Autodesk Inventor part; units mm, degrees
ref_plane "Work Plane1" through (49.8, -24.875, -24.875) normal (1, 0, 0) x (0, 1, 0)
ref_plane "YZ Plane" through (0, 0, 0) normal (1, 0, 0) x (0, 1, 0)
ref_plane "XZ Plane" through (0, 0, 0) normal (0, 1, 0) x (-1, 0, 0)
sketch "Sketch1" plane through (0, 0, 0) normal (1, 0, 0) x (0, 1, 0)
  circle A0 centre (-21.9, 21.9) radius 1.875
  circle A1 centre (21.9, -21.9) radius 1.875
  circle A2 centre (-21.9, -21.9) radius 1.875
  circle A3 centre (21.9, 21.9) radius 1.875
  circle A4 centre (20.8, -14.4) radius 2.0734
  circle A5 centre (-20.8, 14.4) radius 2.0734
  circle A6 centre (-20.8, -14.4) radius 2.0734
  circle A7 centre (-14.4, -20.8) radius 2.0734
  line L0 (17.05, 17.05) -> (-17.05, 17.05)
  line L1 (17.05, -17.05) -> (17.05, 17.05)
  line L2 (-17.05, -17.05) -> (17.05, -17.05)
  line L3 (-17.05, 17.05) -> (-17.05, -17.05)
  circle A8 centre (14.4, -20.8) radius 2.0734
  circle A9 centre (20.8, 14.4) radius 2.0734
  circle A10 centre (-14.4, 20.8) radius 2.0734
  circle A11 centre (14.4, 20.8) radius 2.0734
  line L4 (24.875, 22.9) -> (24.875, -22.9)
  arc A12 (24.875, 22.9) -> (22.9, 24.875) centre (22.9, 22.9) ccw
  line L5 (-22.9, 24.875) -> (22.9, 24.875)
  arc A13 (-22.9, 24.875) -> (-24.875, 22.9) centre (-22.9, 22.9) ccw
  line L6 (-24.875, -22.9) -> (-24.875, 22.9)
  arc A14 (-24.875, -22.9) -> (-22.9, -24.875) centre (-22.9, -22.9) ccw
  line L7 (22.9, -24.875) -> (-22.9, -24.875)
  arc A15 (22.9, -24.875) -> (24.875, -22.9) centre (22.9, -22.9) ccw
  arc A16 (-24.625, -22.9) -> (-22.9, -24.625) centre (-22.9, -22.9) ccw
  line L8 (-24.625, -22.9) -> (-24.625, 22.9)
  arc A17 (-22.9, 24.625) -> (-24.625, 22.9) centre (-22.9, 22.9) ccw
  line L9 (-22.9, 24.625) -> (22.9, 24.625)
  arc A18 (24.625, 22.9) -> (22.9, 24.625) centre (22.9, 22.9) ccw
  line L10 (24.625, 22.9) -> (24.625, -22.9)
  arc A19 (22.9, -24.625) -> (24.625, -22.9) centre (22.9, -22.9) ccw
  line L11 (22.9, -24.625) -> (-22.9, -24.625)
  point P0 (0, 0)
  dimension "d0" = 0.25
ref_plane "Work Plane1" through (49.8, -24.875, -24.875) normal (1, 0, 0) x (0, 1, 0)
extrude "Extrusion1" add sketch "Sketch1" along normal blind 2.5 from surface at 49.8 contours A0 | A1 | A2 | A3 | A4 | A5 | A6 | A7 | L1 L2 L3 L0 | A8 | A9 | A10 | A11 | L8 A17 L9 A18 L10 A19 L11 A16
sketch "Sketch2" plane through (52.3, -22.9, -24.625) normal (1, 0, 0) x (0, 0, -1)
  circle A0 centre (-46.525, 1) radius 1.875
  circle A1 centre (-2.725, 44.8) radius 1.875
  circle A2 centre (-2.725, 1) radius 1.875
  circle A3 centre (-46.525, 44.8) radius 1.875
  circle A4 centre (-10.225, 43.7) radius 2.0734
  circle A5 centre (-39.025, 2.1) radius 2.0734
  circle A6 centre (-10.225, 2.1) radius 2.0734
  circle A7 centre (-3.825, 8.5) radius 2.0734
  line L0 (-41.675, 39.95) -> (-41.675, 5.85)
  line L1 (-7.575, 39.95) -> (-41.675, 39.95)
  line L2 (-7.575, 5.85) -> (-7.575, 39.95)
  line L3 (-41.675, 5.85) -> (-7.575, 5.85)
  circle A8 centre (-3.825, 37.3) radius 2.0734
  circle A9 centre (-39.025, 43.7) radius 2.0734
  circle A10 centre (-45.425, 8.5) radius 2.0734
  circle A11 centre (-45.425, 37.3) radius 2.0734
  line L4 (-47.525, 47.775) -> (-1.725, 47.775)
  arc A12 (-47.525, 47.775) -> (-49.5, 45.8) centre (-47.525, 45.8) ccw
  line L5 (-49.5, 0) -> (-49.5, 45.8)
  arc A13 (-49.5, 0) -> (-47.525, -1.975) centre (-47.525, 0) ccw
  line L6 (-1.725, -1.975) -> (-47.525, -1.975)
  arc A14 (-1.725, -1.975) -> (0.25, 0) centre (-1.725, 0) ccw
  line L7 (0.25, 45.8) -> (0.25, 0)
  arc A15 (0.25, 45.8) -> (-1.725, 47.775) centre (-1.725, 45.8) ccw
  line L8 (-41.6, 39.875) -> (-41.6, 5.925)
  line L9 (-41.6, 5.925) -> (-7.65, 5.925)
  line L10 (-7.65, 5.925) -> (-7.65, 39.875)
  line L11 (-7.65, 39.875) -> (-41.6, 39.875)
  line L12 (-40.35, 38.625) -> (-40.35, 7.175)
  line L13 (-40.35, 7.175) -> (-8.9, 7.175)
  line L14 (-8.9, 7.175) -> (-8.9, 38.625)
  line L15 (-8.9, 38.625) -> (-40.35, 38.625)
  dimension "d16" = 0.075
  dimension "d17" = 1.25
extrude "Extrusion2" add sketch "Sketch2" against normal blind 2.5 from surface at -2.5 contours L11 L10 L9 L8
properties part number "Cover Top (Normal) Proto"
Input: part model. Units: mm. Frame: model coordinates. A direction names the side the tool comes from. Give positions to 0.01 mm unless a question says otherwise; leave off trailing zeros. Order: outer loops, then holes, each group sorted by start corner. A loop starts at its lowest first (then second) coordinate and runs counter-clockwise, first axis right, second up. Notation, with made-up numbers: (6, 11.5) - (37, 11.5) arc R16 cw to (37, 15.5) - close; hole circle Ø1 at (25, 4). An arc over 180 degrees is marked (long way). Write each question's results on one line, items separated by ' | '.
Item 1: Contact query for flat-ended pins moving along their axis: pin 1 Ø15 at (y, z) = (-4.5, -1) entering from -X; pin 2 Ø2 at (x, z) = (48, 4.5) entering from -Y (3 decimals); pin 3 Ø0.8 at (x, z) = (48.5, 3) entering from +Y (3 decimals); pin 4 Ø3 at (x, y) = (49, 0) entering from +Z (3 decimals). Output: stop coordinate, or through.
A:
pin 1: stops at x = 49.8 | pin 2: stops at y = -16.975 | pin 3: stops at y = 16.975 | pin 4: stops at z = 24.625
Item 2: Draft query along Y for faces 5 (the flat face through (51, 24.625, 0)), 6 (the flat face through (49, 0, 16.975)), 7 (the flat face through (49.8, 0, 0)). Return one class per face: released by +Y, released by -Y, zero draft, split by the parting line, or undercut.
A:
face 5: released by +Y | face 6: zero draft | face 7: undercut
Item 3: Material intervals for line 1 along Y through (x, z) = (47.8, 12.5) (3 decimals); line 2 along X through (y, z) = (11, 0), sorted ascending.
A:
line 1: y = -16.975 to -15.725, 15.725 to 16.975 | line 2: x = 49.8 to 52.3
Item 4: Section A-A (y = 1.5). Return loops of the section in (x, z) (3 decimals).
A:
outline: (47.3, -16.975) - (49.8, -16.975) - (49.8, -24.625) - (52.3, -24.625) - (52.3, 24.625) - (49.8, 24.625) - (49.8, 16.975) - (47.3, 16.975) - (47.3, 15.725) - (49.8, 15.725) - (49.8, -15.725) - (47.3, -15.725) - close
Item 5: Section B-B (x = 48.75). Return loops of the section in (y, z) (3 decimals), and give its area (4 significant figures).
A:
outline: (-16.975, -16.975) - (16.975, -16.975) - (16.975, 16.975) - (-16.975, 16.975) - close; hole (-15.725, -15.725) - (15.725, -15.725) - (15.725, 15.725) - (-15.725, 15.725) - close | area: 163.5 mm^2
Item 6: Section D-D (y = -18). Return loops of the section in (x, z) (3 decimals), and give its area (3 significant figures).
A:
outline: (49.8, -24.625) - (52.3, -24.625) - (52.3, 24.625) - (49.8, 24.625) - close | area: 123 mm^2
Item 7: Access query for faces 1 (the flat face through (51, -24.625, 0)), 2 (the flat face through (49, 16.975, 0)), 3 (the flat face through (49, -16.975, 0)), 4 (the flat face through (49, 0, -15.725)). Directions: +Z, -Z, +X, -X, +Y, -Y. A direction counts if a zero-diameter tool reaches every point of the face in a straight line with its end or side. Return the directions, or none.
A:
face 1: +Z, -Z, +X, -X, -Y | face 2: +Z, -Z, -X, +Y | face 3: +Z, -Z, -X, -Y | face 4: -X
